from build123d import *
from OCP.BRepAlgoAPI import BRepAlgoAPI_Cut
from OCP.TopTools import TopTools_ListOfShape

# Parameters (mm, degrees)
BOSS_EXTRUDE1_DEPTH = 1.5875
SKETCH2_R           = 13.081
CUT_EXTRUDE1_DEPTH  = 117.6782
CUT_EXTRUDE2_REACH  = 864.179
SKETCH3_R           = 13.081
SKETCH7_RX          = 13.456940142
SKETCH7_RY          = 13.355964413
CUT_EXTRUDE5_DEPTH  = 523.187556795
SKETCH9_RX          = 13.445467768
SKETCH9_RY          = 13.391794978
CUT_EXTRUDE6_DEPTH  = 523.187556795
SKETCH10_RX         = 13.456940142
SKETCH10_RY         = 13.397800125
CUT_EXTRUDE7_DEPTH  = 523.187556799
CUT_EXTRUDE8_REACH  = 572.923
SKETCH11_R          = 13.081
SKETCH19_RX         = 13.223312173
SKETCH19_RY         = 13.081030132
CUT_EXTRUDE13_DEPTH = 523.187556806
MIRROR1_START       = 1016
MIRROR1_DEPTH       = 5
FILLET1_START       = 1017.2446
FILLET1_DEPTH       = 3.175
CUT_EXTRUDE14_DEPTH = 523.187556802


with BuildPart() as part:
    # Sketch1 → Boss-Extrude1 (new, symmetric)
    with BuildSketch(Plane(origin=(1018.8321, 0, 0), x_dir=(0, 0, -1), z_dir=(1, 0, 0))):
        Polygon((-44.943661408, 213.749166265), (-98.918661408, 213.749166265), (-98.918661408, 67.699166265), (-359.268661408, 67.699166265), (-359.268661408, 245.499166265), (-460.868661408, 244.475), (-460.868661408, 66.675), (-460.868661408, 1.7907), (-384.668661408, 1.7907), (-384.668661408, -1.7907), (-460.868661408, -1.7907), (-460.868661408, -66.675), (-460.868661408, -243.450833735), (-359.268661408, -243.450833735), (-359.268661408, -65.650833735), (-98.918661408, -65.650833735), (-98.918661408, -211.700833735), (-44.943661408, -211.700833735), (-44.943661408, -66.675), (0, -66.675), (0, -193.675), (139.7, -193.675), (139.7, -92.075), (98.24556941, -92.075), (98.24556941, -88.9), (139.7, -88.9), (139.7, 88.9), (98.24556941, 88.9), (98.24556941, 92.075), (139.7, 92.075), (139.7, 193.675), (0, 193.675), (0, 66.675), (-44.943661408, 66.675), align=None)
        with BuildLine():
            add(Edge.make_bspline(
                [(21.556758498, -44.857666301), (-0.366066463, -43.052189708), (9.01360266, -63.161093791), (18.393271782, -83.269997873), (30.936427621, -64.966570384), (43.479583459, -46.663142895), (21.556758498, -44.857666301)],
                knots=[0, 0, 0, 2.094395102, 2.094395102, 4.188790205, 4.188790205, 6.283185307, 6.283185307, 6.283185307], degree=2, weights=[1, 0.5, 1, 0.5, 1, 0.5, 1]))
        make_face(mode=Mode.SUBTRACT)
        with BuildLine():
            add(Edge.make_bspline(
                [(21.556758498, 44.857666301), (43.479583459, 46.663142895), (30.936427621, 64.966570384), (18.393271782, 83.269997873), (9.01360266, 63.161093791), (-0.366066463, 43.052189708), (21.556758498, 44.857666301)],
                knots=[0, 0, 0, 2.094395102, 2.094395102, 4.188790205, 4.188790205, 6.283185307, 6.283185307, 6.283185307], degree=2, weights=[1, 0.5, 1, 0.5, 1, 0.5, 1]))
        make_face(mode=Mode.SUBTRACT)
    extrude(amount=BOSS_EXTRUDE1_DEPTH, both=True)

    # Sketch2 → Cut-Extrude1 (cut)
    with BuildSketch(Plane(origin=(1134.9228, 136.166603714, 0), x_dir=(0, 0, 1), z_dir=(-1, 0, 0))):
        Circle(SKETCH2_R)
    extrude(amount=CUT_EXTRUDE1_DEPTH, mode=Mode.SUBTRACT)

    # Cut-Extrude2: up to this plane
    cut_extrude2_end = Plane(origin=(1017.2446, 0, 0), z_dir=(1, 0, 0))
    # Sketch3 → Cut-Extrude2 (cut, up to the surface)
    with BuildSketch(Plane(origin=(1630.2228, 139.7, 330.2), x_dir=(0.2050222561191695, -0.014387526745204883, 0.9786515588144545), z_dir=(-0.9762506927412319, 0.06850882054324438, 0.20552646162973348)), mode=Mode.PRIVATE) as cut_extrude2_sk1:
        Circle(SKETCH3_R)
    cut_extrude2_tool1 = split(extrude(cut_extrude2_sk1.sketch, amount=CUT_EXTRUDE2_REACH, mode=Mode.PRIVATE), bisect_by=cut_extrude2_end, keep=Keep.BOTH, mode=Mode.PRIVATE)
    add(cut_extrude2_tool1.solids().sort_by_distance((1630.2228, 139.7, 330.2))[0], mode=Mode.SUBTRACT)

    # Sketch7 → Cut-Extrude5 (cut, through all)
    with BuildSketch(Plane.ZY.offset(-1017.2446)):
        with Locations(Location((458.579621053, 182.493207018), (0, 0, 80.206302576))):
            Ellipse(SKETCH7_RX, SKETCH7_RY)
    extrude(amount=-CUT_EXTRUDE5_DEPTH, mode=Mode.SUBTRACT)

    # Sketch9 → Cut-Extrude6 (cut, through all)
    with BuildSketch(Plane(origin=(1020.4196, 0, 0), x_dir=(0, 0, -1), z_dir=(1, 0, 0))):
        with Locations(Location((-458.579621053, 182.493207018), (0, 0, -99.802136374))):
            Ellipse(SKETCH9_RX, SKETCH9_RY)
    extrude(amount=-CUT_EXTRUDE6_DEPTH, mode=Mode.SUBTRACT)

    # Sketch10 → Cut-Extrude7 (cut, through all)
    with BuildSketch(Plane.ZY.offset(-1017.2446)):
        with Locations(Location((458.579621053, 182.493207018), (0, 0, 80.206302562))):
            Ellipse(SKETCH10_RX, SKETCH10_RY)
    extrude(amount=-CUT_EXTRUDE7_DEPTH, mode=Mode.SUBTRACT)

    # Cut-Extrude8: up to this plane
    cut_extrude8_end = Plane(origin=(1017.2446, 0, 0), z_dir=(1, 0, 0))
    # Sketch11 → Cut-Extrude8 (cut, up to the surface)
    with BuildSketch(Plane(origin=(1134.9228, 182.523820118, 99.41306), x_dir=(0.0021298200845781975, 1.9540206598432437e-06, -0.9999977319287225), z_dir=(0.9999973110652725, 0.0009174556197295962, 0.0021298209809440367)), mode=Mode.PRIVATE) as cut_extrude8_sk1:
        Circle(SKETCH11_R)
    cut_extrude8_tool1 = split(extrude(cut_extrude8_sk1.sketch, amount=-CUT_EXTRUDE8_REACH, mode=Mode.PRIVATE), bisect_by=cut_extrude8_end, keep=Keep.BOTH, mode=Mode.PRIVATE)
    add(cut_extrude8_tool1.solids().sort_by_distance((1134.9228, 182.52382, 99.41306))[0], mode=Mode.SUBTRACT)


with BuildPart() as cut_extrude13_tool:
    # Sketch19 → Cut-Extrude13 (new, through all)
    with BuildSketch(Plane.ZY.offset(-1017.2446)):
        with Locations(Location((99.162425827, 182.415855302), (0, 0, 91.056275717))):
            Ellipse(SKETCH19_RX, SKETCH19_RY)
    extrude(amount=-CUT_EXTRUDE13_DEPTH)


with BuildPart() as part_1:
    add(part.part)

    # Cut-Extrude13: cut by cut_extrude13_tool, with a tolerance
    cut_extrude13_stock = TopTools_ListOfShape()
    cut_extrude13_stock.Append(part_1.part.wrapped)
    cut_extrude13_tools = TopTools_ListOfShape()
    cut_extrude13_tools.Append(cut_extrude13_tool.part.wrapped)
    cut_extrude13_cut = BRepAlgoAPI_Cut()
    cut_extrude13_cut.SetArguments(cut_extrude13_stock)
    cut_extrude13_cut.SetTools(cut_extrude13_tools)
    cut_extrude13_cut.SetFuzzyValue(0.00001)
    cut_extrude13_cut.Build()
    add(Compound.cast(cut_extrude13_cut.Shape()).solids(), mode=Mode.REPLACE)

    # Mirror1: read off the stored shape, not the designer's step
    # Mirror1 outline → Mirror1 (cut)
    with BuildSketch(Plane.YZ.offset(MIRROR1_START)):
        with BuildLine():
            add(Edge.make_bspline(
                [(-184.772187594, 445.377072218), (-192.867269369, 446.753422284), (-195.322490897, 454.559086735)],
                knots=[1.911546311, 1.911546311, 1.911546311, 3.008453954, 3.008453954, 3.008453954], degree=2, weights=[1, 0.85333167, 1]))
            add(Edge.make_bspline(
                [(-184.772187594, 445.377072218), (-165.948609057, 442.127807973), (-169.239167993, 460.868661408)],
                knots=[1.570796327, 1.570796327, 1.570796327, 3.484936818, 3.484936818, 3.484936818], degree=2, weights=[1, 0.575917551, 1]))
            Line((-169.239167993, 460.868661408), (-195.754033999, 460.868661411))
            add(Edge.make_bspline(
                [(-195.754033999, 460.868661411), (-196.307414343, 457.662828466), (-195.322490897, 454.559086735)],
                knots=[0, 0, 0, 0.476417942, 0.476417942, 0.476417942], degree=2, weights=[1, 0.971762149, 1]))
        make_face()
        with BuildLine():
            Line((-169.194986689, 98.918661408), (-195.636920453, 98.918661408))
            add(Edge.make_bspline(
                [(-195.636920453, 98.918661408), (-195.40023147, 86.081347081), (-182.421128696, 86.081347081), (-169.442025922, 86.081347081), (-169.194986689, 98.918661408)],
                knots=[0, 0, 0, 1.552160362, 1.552160362, 3.104320723, 3.104320723, 3.104320723], degree=2, weights=[1, 0.713664798, 1, 0.713664798, 1]))
        make_face()
        with BuildLine():
            Line((-123.085603714, 0), (-149.247603714, 0))
            ThreePointArc((-149.247603714, 0), (-136.166603714, -13.081), (-123.085603714, 0))
        make_face()
    extrude(amount=MIRROR1_DEPTH, mode=Mode.SUBTRACT)

    # Fillet1: read off the stored shape, not the designer's step
    # Fillet1 outline → Fillet1 (add)
    with BuildSketch(Plane.YZ.offset(FILLET1_START)):
        with BuildLine():
            ThreePointArc((93.099166265, 98.918661408), (75.138654023, 106.358149166), (67.699166265, 124.318661408))
            Line((67.699166265, 124.318661408), (67.699166265, 98.918661408))
            Line((67.699166265, 98.918661408), (93.099166265, 98.918661408))
        make_face()
        with BuildLine():
            ThreePointArc((67.699166265, 333.868661408), (75.138654023, 351.82917365), (93.099166265, 359.268661408))
            Line((93.099166265, 359.268661408), (67.699166265, 359.268661408))
            Line((67.699166265, 359.268661408), (67.699166265, 333.868661408))
        make_face()
        with BuildLine():
            ThreePointArc((-91.050833735, 359.268661408), (-73.090321493, 351.82917365), (-65.650833735, 333.868661408))
            Line((-65.650833735, 333.868661408), (-65.650833735, 359.268661408))
            Line((-65.650833735, 359.268661408), (-91.050833735, 359.268661408))
        make_face()
        with BuildLine():
            Line((-65.650833735, 98.918661408), (-65.650833735, 124.318661408))
            ThreePointArc((-65.650833735, 124.318661408), (-73.090321493, 106.358149166), (-91.050833735, 98.918661408))
            Line((-91.050833735, 98.918661408), (-65.650833735, 98.918661408))
        make_face()
        with BuildLine():
            ThreePointArc((-66.84434752, 22.471830704), (-75.181443538, 6.43245535), (-92.075, 0))
            Line((-92.075, 0), (-66.675, 0))
            Line((-66.675, 0), (-66.675, 44.943661408))
            Line((-66.675, 44.943661408), (-92.075, 44.943661408))
            ThreePointArc((-92.075, 44.943661408), (-75.181443538, 38.511206058), (-66.84434752, 22.471830704))
        make_face()
        with BuildLine():
            ThreePointArc((92.075, 0), (75.181443538, 6.43245535), (66.84434752, 22.471830704))
            ThreePointArc((66.84434752, 22.471830704), (75.181443538, 38.511206058), (92.075, 44.943661408))
            Line((92.075, 44.943661408), (66.675, 44.943661408))
            Line((66.675, 44.943661408), (66.675, 0))
            Line((66.675, 0), (92.075, 0))
        make_face()
    extrude(amount=FILLET1_DEPTH)

    # Sketch20 → Cut-Extrude14 (cut, through all)
    with BuildSketch(Plane(origin=(1020.4196, 0, 0), x_dir=(0, 0, -1), z_dir=(1, 0, 0))):
        with BuildLine():
            Line((-54.468661408, 140.709369646), (-44.943661408, 140.709369646))
            Line((-44.943661408, 140.709369646), (-44.943661408, 175.649166265))
            Line((-44.943661408, 175.649166265), (-54.468661408, 175.649166265))
            ThreePointArc((-54.468661408, 175.649166265), (-71.938559718, 158.179267956), (-54.468661408, 140.709369646))
        make_face()
    cut_extrude14 = extrude(amount=-CUT_EXTRUDE14_DEPTH, mode=Mode.SUBTRACT)

    # Mirror2: Cut-Extrude14 across plane
    add(cut_extrude14.mirror(Plane.ZX), mode=Mode.SUBTRACT)


solid = part_1.part
CAD build for the part. Positions are in the model's coordinates, mm. A direction names the side the tool comes from. Round coordinates to 2 decimals unless told otherwise and drop trailing zeros. Write each loop counter-clockwise with the first axis right and the second up, starting at its lowest first coordinate (ties: lowest second). Pieces come first, ordered by that corner, then holes. Notation, with made-up numbers: M 67,19.5 L 121,19.5 A34 cw 121,55.5 Z; hole C -35.75,46.25 d4. An arc over 180 degrees is marked long. Use a Markdown table: item, result. Add a question column.
1. Pull direction Z, two halves, no side cores. Call faces 1 (the face through (1018.81, 74.99, 38.34)), 2 (the face through (1017.245, -2, 165)), 3 (the face through (1018.81, -73.289, 352.026)): released by +Z, released by -Z, zero draft, split by the parting line, or undercut.
2. Drill centre lines: probe 1 along Y at (x, z) = (1017.5, -19) (3 decimals); probe 2 along Z at (x, y) = (1017.45, 118); probe 3 along Z at (x, y) = (1019.6, -91). Where is each one in solid material? Low to high.
3. 3-axis set-ups, long thin cutter, end or side, ignore diameter. For faces 4 (the face through (1020.42, -2, 165)), 5 (the face through (1018.81, -74.989, 6.606)), 6 (the face through (1018.8, 75.3, 106.2)), 7 (the face through (1018.854, -158.563, 71.934)): which of +Z, -Z, +X, -X, +Y, -Y reach the whole face in a straight line?
4. Slice it at B-B on x = 1018.25. Give the number of separate pieces and of enclosed holes in the cut face, then the cut area to 3 significant figures.
5. Flat gauge pins, fed straight in: P1, Ø1.5, axis at x = 1017.5, z = -40.5, coming from the +Y side (3 decimals); P2, Ø1.6, axis at x = 1019, z = 48.5, coming from the +Y side; P3, Ø1, axis at x = 1018.5, z = 246, coming from the -Y side. Where does each tip first touch, or does it go through?
6. Slice it at C-C on z = 143. Give the cut face in (x, y).
7. Slice it at A-A on z = -54.5. Give the cut face in (x, y) (3 decimals).
Reply:
| question | item | result |
|---|---|---|
| 1 | face 1 | undercut |
| 1 | face 2 | zero draft |
| 1 | face 3 | undercut |
| 2 | probe 1 | y = -193.675 to -70.421, -44.908 to 44.908, 70.421 to 193.675 |
| 2 | probe 2 | z = -139.7 to 0, 44.94 to 98.92, 359.27 to 460.87 |
| 2 | probe 3 | z = -98.25 to 0.02, 44.92 to 98.92, 359.27 to 460.87 |
| 3 | face 4 | +Z, -Z, +X, +Y, -Y |
| 3 | face 5 | +X, -X, -Y |
| 3 | face 6 | +X, -X, +Y |
| 3 | face 7 | +X, -X |
| 4 | separate pieces | 1 |
| 4 | enclosed holes | 2 |
| 4 | area | 164,000 mm^2 |
| 5 | P1 | stops at y = 193.675 |
| 5 | P2 | stops at y = 213.75 |
| 5 | P3 | stops at y = -65.65 |
| 6 | outline | M 1017.24,-65.65 L 1020.42,-65.65 L 1020.42,67.7 L 1017.24,67.7 Z |
| 7 | outline | M 1017.245,-193.675 L 1020.42,-193.675 L 1020.42,193.675 L 1017.245,193.675 Z |
